Verification items for the finished model (mm, model axes). Face numbers are marked on the shaded views. A direction names the side the tool comes from. Round coordinates to 2 decimals unless told otherwise and drop trailing zeros. Write each loop counter-clockwise with the first axis right and the second up, starting at its lowest first coordinate (ties: lowest second). Pieces come first, ordered by that corner, then holes. Notation, with made-up numbers: M 22.25,-19 L 41.25,-19 A9 ccw 41.25,-3 Z; hole C 25.5,-9.75 d6. An arc over 180 degrees is marked long. One line per item, written item: value. Start each with the question number.
Item 1: Section check A-A, the plane x = 74.5. Record the cut outline in (y, z), then the cut area to 3 significant figures.
Item 2: Tool access check on the marked faces 4 and 5. Record the directions out of +Z, -Z, +X, -X, +Y, -Y that give a thin tool (end or side, any length) a straight path to the whole face; none if there is none.
Item 3: Draft check along Y on the marked faces 1, 2 and 3. Enter one of: +Y half, -Y half, draft (parallel to the pull), parting line (faces both ways), or undercut.
Item 4: Gauge pin test, flat ends, axial feed: pin 1 (3.5 mm diameter, centred on y = -3.5, z = 6.5, fed in from +X); pin 2 (1.5 mm diameter, centred on x = -104, z = 15, fed in from -Y); pin 3 (6.5 mm diameter, centred on y = -7, z = 6, fed in from -X); pin 4 (3 mm diameter, centred on x = -101, y = 5, fed in from +Z). Record the tip position at first contact, or that the pin passes through.
Item 5: Section check B-B, the plane y = 5.5. Record the cut outline in (x, z).
Item 6: Thickness scan on probe 1 along Y at (x, z) = (80, 15.75); probe 2 along Y at (x, z) = (-18, 1.5); probe 3 along X at (y, z) = (-6, 4). Record the ranges inside material, lowest first. Write a range as from..to.
Item 7: Section check C-C, the plane z = 14.75. Record the cut outline in (x, y), then the cut area to 3 significant figures.
Item 8: Section check D-D, the plane x = -63. Record the cut outline in (y, z), then the cut area to 3 significant figures.
from build123d import *

# Parameters (mm, degrees)
F2_W     = 0.8
F2_H     = 7.4
F2_W_2   = 121
F2_H_2   = 13.2
F3_DEPTH = 17.8
F4_T     = -0.8


# Not quite as in the source:
# - a shell that OpenCascade refuses in one call is made with other operations: the cavity is built on its own and cut out


with BuildPart() as f3:
    # F2 (on Top) → F3 (new body)
    with BuildSketch(Plane.XY):
        Polygon((-135.5, 9), (-135.5, 8.2), (-134.7, 8.2), (158.7, 8.2), (159.5, 8.2), (159.5, 9), align=None)
        with Locations((159.1, 4.5)):
            Rectangle(F2_W, F2_H)
        with Locations((-135.1, 4.5)):
            Rectangle(F2_W, F2_H)
        with Locations((60.5, -6.6)):
            Rectangle(F2_W_2, F2_H_2)
        Polygon((-135.5, 0), (0, 0), (121, 0), (159.5, 0), (159.5, 0.8), (158.7, 0.8), (-134.7, 0.8), (-135.5, 0.8), align=None)
    extrude(amount=F3_DEPTH)

    # F4: a shell. OpenCascade refuses it in one call, so the cavity is built on its own and cut out:
    # the body offset inwards by the wall thickness, plus a prism from it out through each open face.
    f4_core = offset(f3.part, amount=F4_T, kind=Kind.INTERSECTION, mode=Mode.PRIVATE)
    f4_exits = [f4_core.faces().sort_by_distance(p)[0] for p in [
        (60.5, -6.2, 17),
    ]]
    add(f4_core, mode=Mode.SUBTRACT)
    extrude(f4_exits, amount=-F4_T, mode=Mode.SUBTRACT)


solid = f3.part
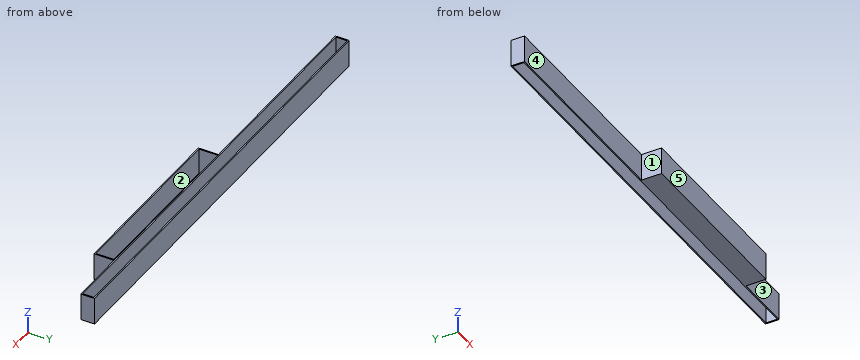
Response values:
1. outline: M -13.2,0 L 0.8,0 L 0.8,17.8 L 0,17.8 L 0,0.8 L -12.4,0.8 L -12.4,17.8 L -13.2,17.8 Z; M 8.2,0 L 9,0 L 9,17.8 L 8.2,17.8 Z
1. area: 52.6 mm2
2. face 4: +Z, -Z, -X, -Y
2. face 5: +Z, -Z, +X, -X, -Y
3. face 1: draft
3. face 2: undercut
3. face 3: -Y half
4. pin 1: stops at x = 121
4. pin 2: stops at y = 0
4. pin 3: stops at x = 0
4. pin 4: passes through
5. outline: M -135.5,0 L -134.7,0 L -134.7,17.8 L -135.5,17.8 Z; M 158.7,0 L 159.5,0 L 159.5,17.8 L 158.7,17.8 Z
6. probe 1: y = -13.2..-12.4, 0..0.8, 8.2..9
6. probe 2: y = 0..0.8, 8.2..9
6. probe 3: x = 0..0.8, 120.2..121
7. outline: M -135.5,0 L 0,0 L 0,-13.2 L 121,-13.2 L 121,0 L 159.5,0 L 159.5,9 L -135.5,9 Z; hole M -134.7,0.8 L 158.7,0.8 L 158.7,8.2 L -134.7,8.2 Z; hole M 0.8,-12.4 L 120.2,-12.4 L 120.2,0 L 0.8,0 Z
7. area: 600 mm2
8. outline: M 0,0 L 0.8,0 L 0.8,17.8 L 0,17.8 Z; M 8.2,0 L 9,0 L 9,17.8 L 8.2,17.8 Z
8. area: 28.5 mm2
